Could you check a few things on this drawing? It's one solid part, dimensions in mm from its lowest x, y, z. Give positions to 0.01 mm unless a question says otherwise; leave off trailing zeros. Loops run counter-clockwise (first coordinate to the right, second up) from the corner with the lowest first, then second, coordinate; pieces in that order, holes last. Notation, with made-up numbers: (-13.5, 2) - (-2.5, 2) arc R20 ccw to (-2.5, 24) - close; hole circle Ø3 at (58, 24.5). An arc over 180 degrees is marked (long way). Return JSON: item names as keys, results as strings. Group by question number.
(1) If we mould it in two halves opening along X, with no side actions, what happens to the marked faces 1, 2, 3 and 4? For each: released by +X, released by -X, zero draft, split by the parting line, or undercut.
(2) If we section it at B-B (z = 54.5): Please give me the cut outline in (x, y), then the cut area to 3 significant figures.
(3) If we section it at D-D (x = 69): Please give me the cut outline in (y, z).
(4) If we section it at A-A (x = 38.5): Please give me the cut outline in (y, z).
(5) If we section it at C-C (y = 9): State how many separate pieces and enclosed holes the cut face has, then the cut area to 3 significant figures.
(6) I need wall thicknesses on probe 1 along Z at (x, y) = (12.5, 12); probe 2 along Z at (x, y) = (26, 4.75); probe 3 along X at (y, z) = (17.25, 25.5). Which ranges of each line are inside material? Lowest first, please. Write a range as [from, to].
(7) For P1, Ø2.5, axis at x = 10.5, z = 78, coming from the +Y side; P2, Ø9.5, axis at x = 19, y = 9, coming from the +Z side; P3, Ø9.5, axis at x = 69, y = 9, coming from the -Z side, each with a flat end and sliding along its axis, tell me the tip position at first contact or that it passes through.
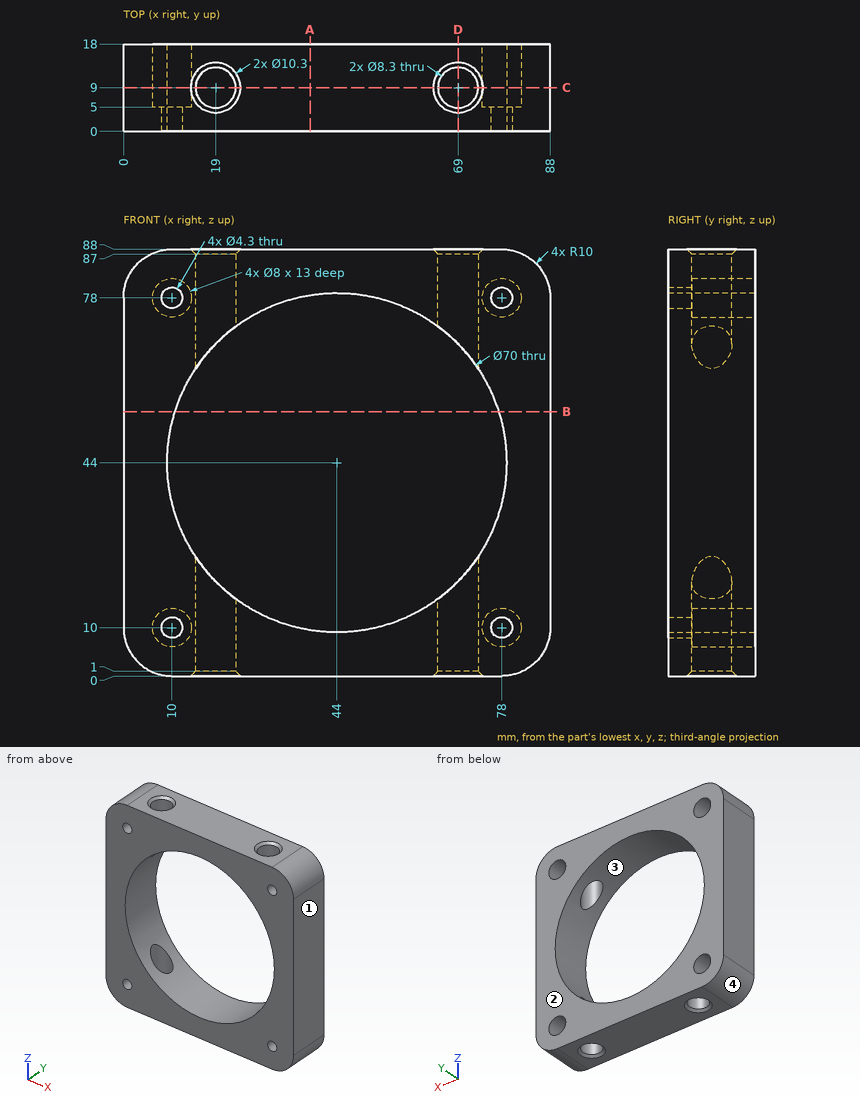
Values:
{
 "1": {"face 1": "released by +X", "face 2": "zero draft", "face 3": "undercut", "face 4": "released by -X"},
 "2": {"outline": "(0, 0) - (10.61, 0) - (10.61, 18) - (0, 18) - close; (77.39, 0) - (88, 0) - (88, 18) - (77.39, 18) - close", "area": "382 mm2"},
 "3": {"outline": "(0, 0) - (3.85, 0) - (4.85, 1) - (4.85, 19.51) - (0, 19.51) - close; (0, 68.49) - (4.85, 68.49) - (4.85, 87) - (3.85, 88) - (0, 88) - close; (13.15, 1) - (14.15, 0) - (18, 0) - (18, 19.51) - (13.15, 19.51) - close; (13.15, 68.49) - (18, 68.49) - (18, 88) - (14.15, 88) - (13.15, 87) - close"},
 "4": {"outline": "(0, 0) - (18, 0) - (18, 9.43) - (0, 9.43) - close; (0, 78.57) - (18, 78.57) - (18, 88) - (0, 88) - close"},
 "5": {"separate pieces": "4", "enclosed holes": "4", "area": "2,950 mm2"},
 "6": {"probe 1": "[0, 6.88], [13.12, 28.74], [59.26, 74.88], [81.12, 88]", "probe 2": "[0, 13.98], [74.02, 88]", "probe 3": "[0, 14.29], [73.71, 88]"},
 "7": {"P1": "through", "P2": "z = 87.6", "P3": "z = 0.4"}
}
